For this review, use the dimensioned drawing (mm, ordinates from the lowest corner) and the shaded views. Give positions to 0.01 mm unless a question says otherwise; leave off trailing zeros. Write each loop counter-clockwise with the first axis right and the second up, starting at its lowest first coordinate (ties: lowest second). Pieces come first, ordered by that corner, then holes. Notation, with made-up numbers: (17.5, 37) -> (49.5, 37) arc R11 ccw to (49.5, 53) -> close; hole circle Ø1 at (36, -8.5). An arc over 180 degrees is marked (long way). Return JSON: item names as keys, results as strings.
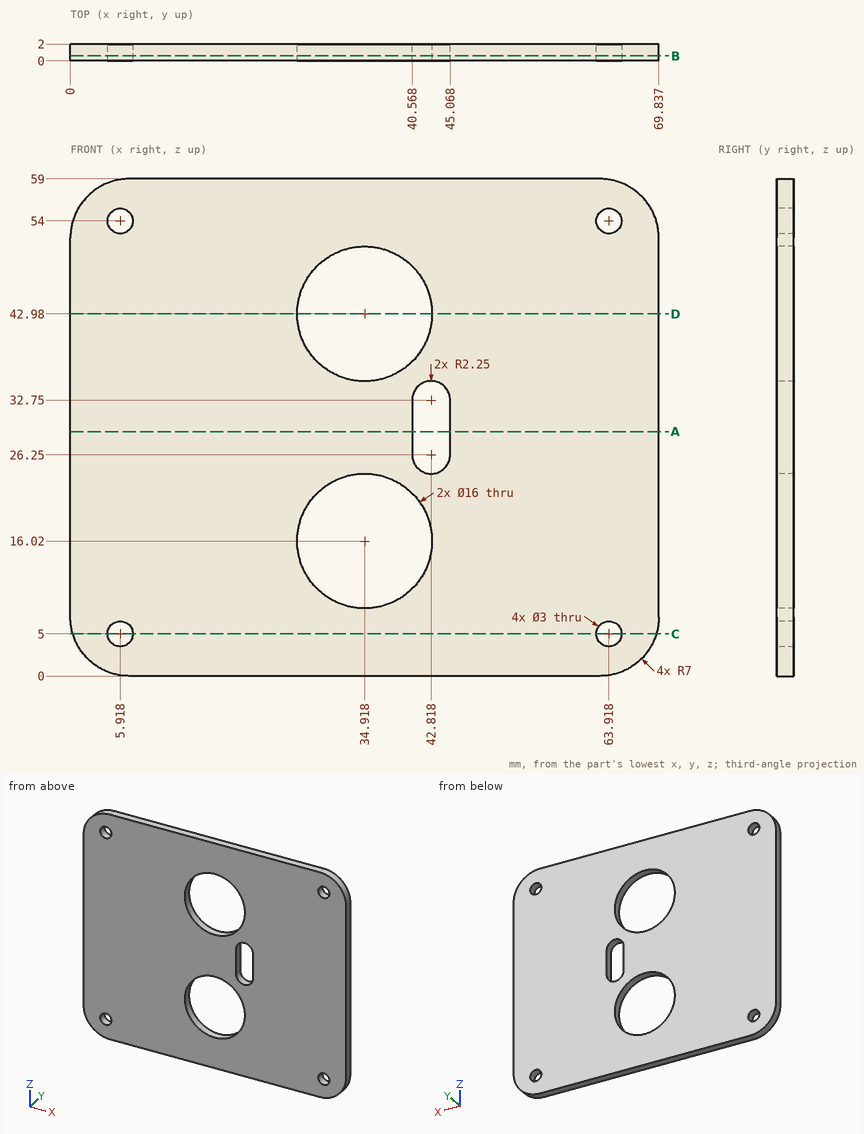
1. Add section A-A, the plane z = 29. State the section outline as (x, y) points, plus the area to 3 significant figures.
Results found:
{"outline": "(0, 0) -> (40.57, 0) -> (40.57, 2) -> (0, 2) -> close; (45.07, 0) -> (69.84, 0) -> (69.84, 2) -> (45.07, 2) -> close", "area": "131 mm²"}
2. To check wall thickness, follow probe 1 along Z at (x, y) = (7, 0.7); probe 2 along Z at (x, y) = (29, 1.8) (1 decimal); probe 3 along X at (y, z) = (1.4, 42.5). State the ranges of each line that lie inside material, in increasing order.
Results found:
{"probe 1": "z = 0 to 3.96, 6.04 to 52.96, 55.04 to 59", "probe 2": "z = 0 to 10.6, 21.4 to 37.6, 48.4 to 59", "probe 3": "x = 0 to 26.93, 42.9 to 69.84"}
3. Add section C-C, the plane z = 5. State the section outline as (x, y) points (1 decimal).
Results found:
{"outline": "(0.3, 0) -> (4.4, 0) -> (4.4, 2) -> (0.3, 2) -> close; (7.4, 0) -> (62.4, 0) -> (62.4, 2) -> (7.4, 2) -> close; (65.4, 0) -> (69.5, 0) -> (69.5, 2) -> (65.4, 2) -> close"}
4. For pin 1 (2.5 mm diameter, centred on x = 5.92, z = 5, fed in from +Y); pin 2 (1 mm diameter, centred on x = 26.5, y = 1.5, fed in from -Z), all flat-tipped, find the tip position at first contact; note any pin that passes through.
Results found:
{"pin 1": "passes through", "pin 2": "stops at z = 0"}
5. Add section D-D, the plane z = 42.98. State the section outline as (x, y) points.
Results found:
{"outline": "(0, 0) -> (26.92, 0) -> (26.92, 2) -> (0, 2) -> close; (42.92, 0) -> (69.84, 0) -> (69.84, 2) -> (42.92, 2) -> close"}
6. Add section B-B, the plane y = 0.6. State the section outline as (x, z) points.
Results found:
{"outline": "(0, 7) arc R7 ccw to (7, 0) -> (62.84, 0) arc R7 ccw to (69.84, 7) -> (69.84, 52) arc R7 ccw to (62.84, 59) -> (7, 59) arc R7 ccw to (0, 52) -> close; hole circle Ø3 at (5.92, 5); hole circle Ø3 at (5.92, 54); hole circle Ø16 at (34.92, 16.02); hole circle Ø16 at (34.92, 42.98); hole (40.57, 26.25) arc R2.25 ccw to (45.07, 26.25) -> (45.07, 32.75) arc R2.25 ccw to (40.57, 32.75) -> close; hole circle Ø3 at (63.92, 5); hole circle Ø3 at (63.92, 54)"}
